Autodesk Inventor part; units mm, degrees
ref_plane "YZ Plane" through (0, 0, 0) normal (1, 0, 0) x (0, 1, 0)
ref_plane "XZ Plane" through (0, 0, 0) normal (0, 1, 0) x (-1, 0, 0)
ref_plane "XY Plane" through (0, 0, 0) normal (0, 0, 1) x (1, 0, 0)
sketch "Sketch1" plane through (0, 0, 0) normal (0, 0, 1) x (1, 0, 0)
  circle A0 centre (0, 0) radius 6.75
  circle A1 centre (0, 0) radius 12
  dimension "d0" = 13.5
  dimension "d1" = 24
extrude "Extrusion1" add sketch "Sketch1" along normal blind 29
sketch "Sketch3" plane through (0, 0, 29) normal (0, 0, 1) x (1, 0, 0)
  circle A0 centre (0, 0) radius 10
  circle A1 centre (0, 0) radius 6.75
  dimension "d7" = 20
extrude "Extrusion3" add sketch "Sketch3" along normal blind 1
sketch "Sketch4" plane through (0, 0, 30) normal (0, 0, 1) x (1, 0, 0)
  line L0 (3.7816, 6.55) -> (7.5633, 0)
  line L1 (7.5633, 0) -> (3.7816, -6.55)
  line L2 (3.7816, -6.55) -> (-3.7816, -6.55)
  line L3 (-3.7816, -6.55) -> (-7.5633, 0)
  line L4 (-7.5633, 0) -> (-3.7816, 6.55)
  line L5 (-3.7816, 6.55) -> (3.7816, 6.55)
  point P0 (0, 0)
  point P1 (0, 0)
  dimension "d10" = 13.1
extrude "Extrusion4" cut sketch "Sketch4" against normal blind 5
sketch "Sketch5" plane through (0, 0, 30) normal (0, 0, 1) x (1, 0, 0)
  line L0 (2, -8.55) -> (-2, -8.55)
  line L1 (-2, -8.55) -> (-2, -4.55)
  line L2 (-2, -4.55) -> (2, -4.55)
  line L3 (2, -4.55) -> (2, -8.55)
  line L4 (3.7816, -6.55) -> (-3.7816, -6.55)
  point P0 (0, 0)
  point P1 (0, -8.55)
  point P2 (-2, -6.55)
  point P3 (0, -6.55)
  dimension "d13" = 4
  dimension "d14" = 4
extrude "Extrusion5" cut sketch "Sketch5" against normal through all
properties part number "Inner Wheel Spacer"
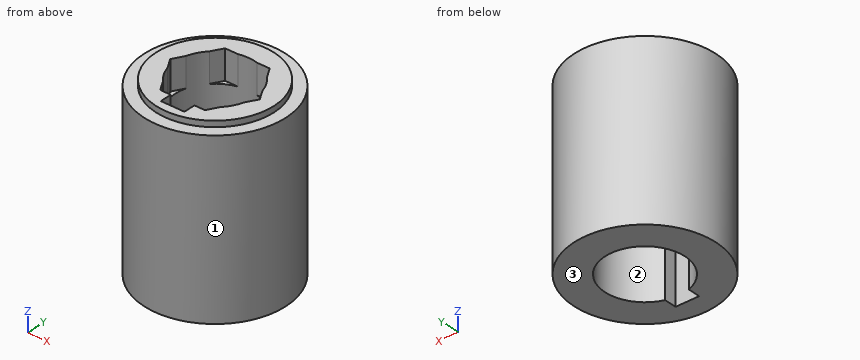
Verification items for the finished model (mm, model axes). Face numbers are marked on the shaded views. Give positions to 0.01 mm unless a question says otherwise; leave off trailing zeros. Loops run counter-clockwise (first coordinate to the right, second up) from the corner with the lowest first, then second, coordinate; pieces in that order, holes last.
1) Draft check along X on the marked faces 1, 2 and 3. Enter one of: pulls with the +X half, pulls with the -X half, needs draft (parallel to the pull), parting line crosses it, or undercut.
2) Sectioned sample at D-D, the plane x = -3. Enter the section's corners in (y, z), then the cut area to 3 significant figures.
3) Thickness scan on line 1 along Y through (x, z) = (0, 19.75); line 2 along Z through (x, y) = (-10, 4.75); line 3 along Y through (x, z) = (6.25, 11.5). Record the ranges inside material, lowest first.
4) Sectioned sample at C-C, the plane z = 15.75. Enter the section's corners in (x, y), then the cut area to 3 significant figures.
5) Sectioned sample at A-A, the plane x = 0. Enter the section's corners in (y, z), then the cut area to 3 significant figures.
6) Sectioned sample at B-B, the plane y = -2.75. Enter the section's corners in (x, z).
7) Depth check by flat-ended pin: pin 1 Ø5 at (x, z) = (9.5, 10.5) entering from -Y; pin 2 Ø5 at (y, z) = (-6, 16) entering from +X; pin 3 Ø2.5 at (x, z) = (2, 28) entering from -Y; pin 4 Ø6 at (y, z) = (2, 20) entering from +X. Enter the tip coordinate at first touch or a pass-through.
Answers:
1. face 1: parting line crosses it
1. face 2: undercut
1. face 3: needs draft
2. outline: (-11.62, 0) - (-6.05, 0) - (-6.05, 25) - (-6.55, 25) - (-6.55, 30) - (-9.54, 30) - (-9.54, 29) - (-11.62, 29) - close; (6.05, 0) - (11.62, 0) - (11.62, 29) - (9.54, 29) - (9.54, 30) - (6.55, 30) - (6.55, 25) - (6.05, 25) - close
2. area: 325 mm2
3. line 1: y = -12 to -8.55, 6.75 to 12
3. line 2: z = 0 to 29
3. line 3: y = -10.24 to -2.55, 2.55 to 10.24
4. outline: circle Ø24 at (0, 0); hole (-2, -8.55) - (2, -8.55) - (2, -6.45) arc R6.75 ccw (long way) to (-2, -6.45) - close
4. area: 302 mm2
5. outline: (-12, 0) - (-8.55, 0) - (-8.55, 30) - (-10, 30) - (-10, 29) - (-12, 29) - close; (6.75, 0) - (12, 0) - (12, 29) - (10, 29) - (10, 30) - (6.75, 30) - close
5. area: 257 mm2
6. outline: (-11.68, 0) - (-6.16, 0) - (-6.16, 30) - (-9.61, 30) - (-9.61, 29) - (-11.68, 29) - close; (6.16, 0) - (11.68, 0) - (11.68, 29) - (9.61, 29) - (9.61, 30) - (6.16, 30) - close
7. pin 1: stops at y = -9.75
7. pin 2: stops at x = 11.48
7. pin 3: stops at y = -11.98
7. pin 4: stops at x = 12
